Source: three-view drawing plus pictorial views. Frame: mm from the lowest corner of the part. A direction names the side the tool comes from. Round coordinates to 2 decimals unless told otherwise and drop trailing zeros. Order: outer loops, then holes, each group sorted by start corner. A loop starts at its lowest first (then second) coordinate and runs counter-clockwise, first axis right, second up. Notation, with made-up numbers: (73, -14) - (97, -14) arc R24 cw to (97, 5) - close; hole circle Ø6 at (-25, 25). An arc over 180 degrees is marked (long way). Use one line per item in the form item = value. Start each with the question number.
Q1. Set-up query: the marked faces 1, 2 and 3. Return all of +Z, -Z, +X, -X, +Y, -Y with unobstructed straight access to the full face (end or side cutting, diameter ignored); none if empty.
Q2. Ray query, line 1 (X direction, y = 15, z = 28) (1 decimal); line 2 (Z direction, x = 28, y = 14.5) (1 decimal); line 3 (X direction, y = 3.5, z = 21.5) (1 decimal). Return the intervals inside material, ascending. Write a range as [from, to].
Q3. Draft query along X for the marked faces 4, 5 and 6. Return one class per face: released by +X, released by -X, zero draft, split by the parting line, or undercut.
Q4. Pin query (flat end, axial travel): pin 1 Ø1.2 at (x, z) = (48, 15) entering from +Y; pin 2 Ø8 at (y, z) = (3, 16.5) entering from -X; pin 3 Ø1.5 at (x, y) = (7, 3.5) entering from -Z. Return the tip coordinate at first contact, or that it passes through.
Q5. Cut plane A-A, the plane y = 11.25. Give the number of separate pieces and of enclosed holes in the cut face, and give its area (3 significant figures).
Q6. Cut plane C-C, the plane z = 39. Return the cut outline in (x, y) (1 decimal).
Q7. Cut plane B-B, the plane x = 34. Return the cut outline in (y, z) (1 decimal).
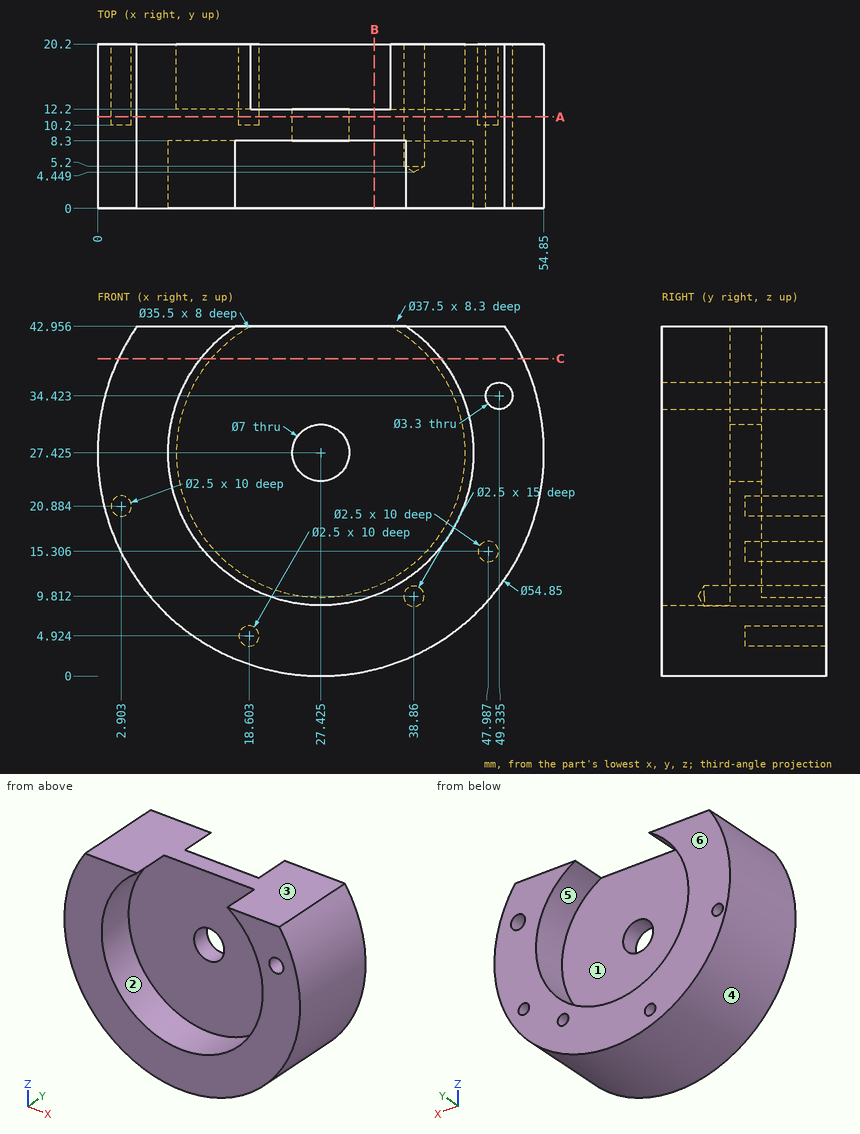
Completed:
q1.face_1 = +Y
q1.face_2 = -Y
q1.face_3 = +Z, +X, -X, +Y, -Y
q2.line_1 = [0, 9.7], [45.2, 54.8]
q2.line_2 = [0, 9.7]
q2.line_3 = [0.6, 9.6], [45.2, 54.2]
q3.face_4 = split by the parting line
q3.face_5 = undercut
q3.face_6 = zero draft
q4.pin_1 = 10.2
q4.pin_2 = 0.89
q4.pin_3 = 8.32
q5.separate_pieces = 1
q5.enclosed_holes = 6
q5.area = 1,920 mm2
q6.outline = (2.6, 0) - (12.7, 0) - (12.7, 8.3) - (42.2, 8.3) - (42.2, 0) - (52.3, 0) - (52.3, 20.2) - (40.9, 20.2) - (40.9, 12.2) - (14, 12.2) - (14, 20.2) - (2.6, 20.2) - close
q7.outline = (0, 0.8) - (20.2, 0.8) - (20.2, 10.9) - (12.2, 10.9) - (12.2, 43) - (8.3, 43) - (8.3, 9.9) - (0, 9.9) - close
